Could you check a few things on this model? Use its own coordinates, in mm. Round coordinates to 2 decimals unless told otherwise and drop trailing zeros. Order: outer loops, then holes, each group sorted by start corner. A loop starts at its lowest first (then second) coordinate and runs counter-clockwise, first axis right, second up. Notation, with made-up numbers: M 11,39.5 L 24,39.5 A17 ccw 24,44.5 Z; hole C -11.5,56 d6. An arc over 180 degrees is marked long. Write each question's results on one line, items separated by ' | '. Start each with the question number.
1. Suppose I cut it at D-D on z = 7.25. Write out the boundary of the cut face in (x, y).
2. Suppose I cut it at B-B on z = 4. Write out the boundary of the cut face in (x, y).
3. I'm going to push a flat-ended pin straight in: pin 1 (1 mm diameter, centred on y = -1.5, z = -5.5, fed in from +X). Where does the tip first touch, or does it pass through?
4. Suppose I cut it at A-A on x = 0.55. Write out the boundary of the cut face in (y, z).
5. Please list where these lines run through material, in increasing order: L1, parallel to Y at x = 0.9, z = -5; L2, parallel to Y at x = 0.15, z = 1.75; L3, parallel to Z at x = 0.05, y = 5.5.
from build123d import *

# Parameters (mm, degrees)
F1_DEPTH = 1.016


with BuildPart() as f1:
    # F0 (on Right) → F1 (new body)
    with BuildSketch(Plane.YZ):
        with BuildLine():
            Line((0, 6.8326), (0, 9.4996))
            ThreePointArc((0, 9.4996), (-6.717232, 6.717232), (-9.4996, 0))
            Line((-9.4996, 0), (-6.8326, 0))
            ThreePointArc((-6.8326, 0), (-4.831378, 4.831378), (0, 6.8326))
        make_face()
        with BuildLine():
            Line((6.8326, 0), (9.4996, 0))
            ThreePointArc((9.4996, 0), (6.717232, 6.717232), (0, 9.4996))
            Line((0, 9.4996), (0, 6.8326))
            ThreePointArc((0, 6.8326), (4.831378, 4.831378), (6.8326, 0))
        make_face()
        with BuildLine():
            ThreePointArc((0, -9.4996), (6.717232, -6.717232), (9.4996, 0))
            Line((9.4996, 0), (6.8326, 0))
            ThreePointArc((6.8326, 0), (4.831378, -4.831378), (0, -6.8326))
            Line((0, -6.8326), (0, -9.4996))
        make_face()
        with BuildLine():
            ThreePointArc((-9.4996, 0), (-6.717232, -6.717232), (0, -9.4996))
            Line((0, -9.4996), (0, -6.8326))
            ThreePointArc((0, -6.8326), (-4.831378, -4.831378), (-6.8326, 0))
            Line((-6.8326, 0), (-9.4996, 0))
        make_face()
    extrude(amount=F1_DEPTH)


solid = f1.part
Filled sheet:
1) outline: M 0,-6.14 L 1.02,-6.14 L 1.02,6.14 L 0,6.14 Z
2) outline: M 0,-8.62 L 1.02,-8.62 L 1.02,-5.54 L 0,-5.54 Z; M 0,5.54 L 1.02,5.54 L 1.02,8.62 L 0,8.62 Z
3) pin 1: passes through
4) outline: M -9.5,0 A9.5 ccw 0,-9.5 A9.5 ccw 9.5,0 A9.5 ccw 0,9.5 A9.5 ccw Z; hole M -6.83,0 A6.83 ccw 0,-6.83 A6.83 ccw 6.83,0 A6.83 ccw 0,6.83 A6.83 ccw Z
5) L1: y = -8.08 to -4.66, 4.66 to 8.08 | L2: y = -9.34 to -6.6, 6.6 to 9.34 | L3: z = -7.75 to -4.05, 4.05 to 7.75
